Autodesk Inventor part; units mm, degrees
ref_plane "YZ Plane" through (0, 0, 0) normal (1, 0, 0) x (0, 1, 0)
ref_plane "XZ Plane" through (0, 0, 0) normal (0, 1, 0) x (-1, 0, 0)
ref_plane "XY Plane" through (0, 0, 0) normal (0, 0, 1) x (1, 0, 0)
sketch "Sketch1" plane through (0, 0, 0) normal (0, 1, 0) x (-1, 0, 0)
  line L0 (10, -45) -> (-10, -45)
  line L1 (-10, -45) -> (-10, 47.1)
  line L2 (-10, 47.1) -> (10, 47.1)
  line L3 (10, 47.1) -> (10, -45)
  point P0 (0, 0)
  dimension "d0" = 20
  dimension "d1" = 92.1
  dimension "d2" = 45
  dimension "d3" = 10
extrude "Plate1" add sketch "Sketch1" along normal blind 1.5
sketch "Sketch2" plane through (0, 0, 0) normal (0, -1, 0) x (1, 0, 0)
  circle A0 centre (0, 42) radius 0.7835
  circle A1 centre (-7, 35) radius 0.7835
  circle A2 centre (0, 28) radius 0.7835
  circle A3 centre (7, 35) radius 0.7835
  circle A4 centre (0, -28) radius 0.7835
  circle A5 centre (-7, -35) radius 0.7835
  circle A6 centre (0, -42) radius 0.7835
  circle A7 centre (7, -35) radius 0.7835
  circle A8 centre (-7, 37) radius 0.7835
  circle A9 centre (0, 30) radius 0.7835
  circle A10 centre (0, 44) radius 0.7835
  circle A11 centre (7, 37) radius 0.7835
  point P0 (0, 0)
hole "Hole1" at (-7, 0, -35) at (7, 0, -35) at (0, 0, -42) at (0, 0, -28) at (7, 0, 37) at (0, 0, 44) at (-7, 0, 37) at (0, 0, 30) direction (0, 1, 0) diameter 2.1 depth 1.5
sketch "Sketch3" plane through (0, 1.5, 0) normal (0, 1, 0) x (1, 0, 0)
  arc A0 (10, 35) -> (-10, 35) centre (0, 35) ccw
  arc A1 (-10, -37.1) -> (10, -37.1) centre (0, -37.1) ccw
  line L0 (-10, 35) -> (-10, -37.1)
  line L1 (10, 35) -> (10, -37.1)
  line L2 (10, 45) -> (10, -47.1)
  line L3 (-10, 45) -> (10, 45)
  line L4 (10, 45) -> (10, -47.1)
  line L5 (10, -47.1) -> (-10, -47.1)
  line L6 (-10, -47.1) -> (-10, 45)
  point P0 (0, 0)
  point P1 (0, 45)
  point P2 (10, 45)
  point P3 (10, 35)
  point P4 (-10, -37.1)
  point P5 (0, -47.1)
  point P6 (10, -37.1)
  point P7 (1.4107, 44.9)
  point P8 (10, 35)
  point P9 (10, -37.1)
  dimension "d12" = 35
  dimension "d13" = 37.1
  dimension "d14" = 10
  dimension "d15" = 10
  dimension "d16" = 10
  dimension "d17" = 20
  dimension "d18" = 92.1
extrude "Extrusion1" cut sketch "Sketch3" against normal blind 10 contours A0 L3 L2 | A0 L6 L3 | L2 L5 A1 | L5 L6 A1
sketch "Sketch4" plane through (0, 0, 0) normal (0, -1, 0) x (1, 0, 0)
  arc A0 (-10, -35) -> (10, -35) centre (0, -35) ccw
  arc A1 (10, 37.1) -> (-10, 37.1) centre (0, 37.1) ccw
  point P0 (0, 0)
hole "Hole2" at (0, 0, 37.1) at (0, 0, -35) direction (0, 1, 0) diameter 7.2 depth 1.5
equation "\"d10\" = Thickness"
equation "\"d26\" = Thickness"
equation "\"d4\" = Thickness"
equation "\"BendReliefWidth\" = Thickness"
equation "\"BendReliefDepth\" = 0.5 * Thickness"
equation "\"CornerReliefSize\" = 4 * Thickness"
equation "\"MinimumRemnant\" = 2 * Thickness"
equation "\"TransitionRadius\" = BendRadius"
equation "\"JacobiRadiusSize\" = BendRadius"
equation "\"GapSize\" = Thickness"
properties part number "axis_10_11-connector_frame" material "Aluminum 6061-AHC"
Build history of the part. All positions in model axes, mm. Give positions to 0.01 mm unless a question says otherwise; leave off trailing zeros. Loops run counter-clockwise (first coordinate to the right, second up) from the corner with the lowest first, then second, coordinate; pieces in that order, holes last.
1) Band-saw the part on A-A on y = 0.9. State how many separate pieces and enclosed holes the cut face has, then the cut area to 3 significant figures.
Values follow:
separate pieces: 1
enclosed holes: 10
area: 1,650 mm2
2) Band-saw the part on D-D on z = 30. List the corners of the cut face in (x, y).
Values follow:
outline: (-10, 0) - (-1.05, 0) - (-1.05, 1.5) - (-10, 1.5) - close; (1.05, 0) - (10, 0) - (10, 1.5) - (1.05, 1.5) - close
3) Two-plate mould, pull along Z, no slides. Class faces 1 (the face through (0, 0, 2)), 2 (the face through (0, 1, -45)), 3 (the face through (-0.05, 0.76, -40.95)), 4 (the face through (-1.081, 0.76, -38.434)): released by +Z, released by -Z, zero draft, split by the parting line, or undercut.
Values follow:
face 1: zero draft
face 2: released by -Z
face 3: undercut
face 4: undercut
4) Probe line 1 along X through (y, z) = (0.75, -35); line 2 along X through (y, z) = (1.1, 30); line 3 along Z through (x, y) = (-7, 0.95). List the from-to ranges inside material, lowest first.
Values follow:
line 1: x = -10 to -8.05, -5.95 to -3.6, 3.6 to 5.95, 8.05 to 10
line 2: x = -10 to -1.05, 1.05 to 10
line 3: z = -42.14 to -36.05, -33.95 to 35.95, 38.05 to 44.24
5) Band-saw the part on C-C on x = 2. List the corners of the cut face in (y, z), then the cut area to 3 significant figures.
Values follow:
outline: (0, -44.8) - (1.5, -44.8) - (1.5, -37.99) - (0, -37.99) - close; (0, -32.01) - (1.5, -32.01) - (1.5, 34.11) - (0, 34.11) - close; (0, 40.09) - (1.5, 40.09) - (1.5, 46.9) - (0, 46.9) - close
area: 120 mm2
6) Band-saw the part on B-B on z = 44. List the corners of the cut face in (x, y), then the cut area to 3 significant figures.
Values follow:
outline: (-7.24, 0) - (-1.05, 0) - (-1.05, 1.5) - (-7.24, 1.5) - close; (1.05, 0) - (7.24, 0) - (7.24, 1.5) - (1.05, 1.5) - close
area: 18.6 mm2
